Autodesk Inventor part; units mm, degrees
ref_plane "YZ Plane" through (0, 0, 0) normal (1, 0, 0) x (0, 1, 0)
ref_plane "XZ Plane" through (0, 0, 0) normal (0, 1, 0) x (-1, 0, 0)
ref_plane "XY Plane" through (0, 0, 0) normal (0, 0, 1) x (1, 0, 0)
sketch "Sketch1" plane through (0, 0, 0) normal (0, 0, 1) x (1, 0, 0)
  arc A0 (1.778, -29.9361) -> (-1.778, -29.9361) centre (0, -31.75) ccw construction
  line L0 (1.778, -29.9361) -> (1.778, -33.5639) construction
  arc A1 (-1.778, -33.5639) -> (1.778, -33.5639) centre (0, -31.75) ccw construction
  line L1 (-1.778, -33.5639) -> (-1.778, -29.9361) construction
  line L2 (1.778, -29.9361) -> (1.778, -33.5639) construction
  line L3 (-1.778, -29.9361) -> (-1.778, -33.5639) construction
  arc A2 (1.778, -29.9361) -> (-1.778, -29.9361) centre (0, -31.75) ccw construction
  arc A3 (-1.778, -33.5639) -> (1.778, -33.5639) centre (0, -31.75) ccw construction
  arc A4 (1.524, -30.0461) -> (-1.524, -30.0461) centre (0, -31.75) ccw
  line L4 (1.524, -30.0461) -> (1.524, -33.4539)
  arc A5 (-1.524, -33.4539) -> (1.524, -33.4539) centre (0, -31.75) ccw
  line L5 (-1.524, -33.4539) -> (-1.524, -30.0461)
  point P0 (0, 0)
  point P1 (0, -34.29)
  point P2 (0, -29.21)
  dimension "d0" = 0.254
extrude "Extrusion1" add sketch "Sketch1" along normal mid plane 36.83
ref_plane "Work Plane1" through (0, 0, 0) normal (0, 0, 1) x (1, 0, 0)
sketch "Sketch2" plane through (0, 0, 0) normal (0, 0, 1) x (1, 0, 0)
  line L0 (31.75, -50.8) -> (-31.75, -50.8)
  line L1 (-31.75, -50.8) -> (-31.75, -12.7)
  line L2 (-31.75, -12.7) -> (31.75, -12.7)
  line L3 (31.75, -12.7) -> (31.75, -50.8)
  line L4 (31.75, -50.8) -> (-31.75, -12.7) construction
  line L5 (-31.75, -50.8) -> (31.75, -12.7) construction
  circle A0 centre (0, -31.75) radius 5.715
  dimension "d5" = 63.5
  dimension "d6" = 38.1
extrude "Extrusion2" add sketch "Sketch2" along normal mid plane 18.669 contours L0 L1 L2 L3 | A0
properties part number "Geared_Motor"
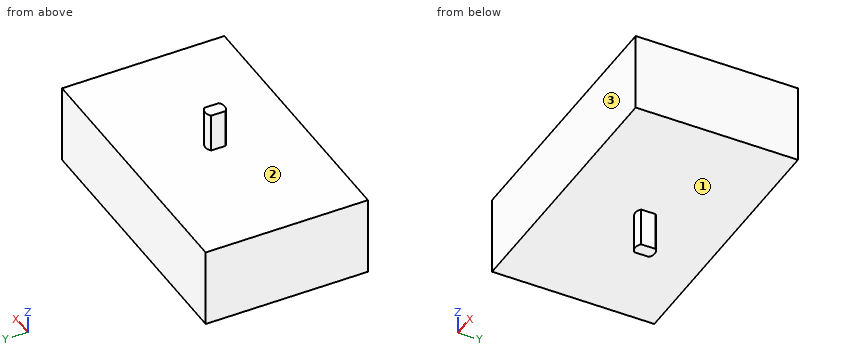
The model under review builds one solid part; all positions refer to its coordinate system, in mm. Face numbers are marked on the shaded views. Round coordinates to 2 decimals unless told otherwise and drop trailing zeros. Write each loop counter-clockwise with the first axis right and the second up, starting at its lowest first coordinate (ties: lowest second). Pieces come first, ordered by that corner, then holes. Notation, with made-up numbers: (37, -39) - (89, -39) arc R34 ccw to (89, -8) - close; hole circle Ø2 at (-38.75, 76.25). An arc over 180 degrees is marked (long way). One line per item, written item: value. Start each with the question number.
1. Consider section B-B on y = -22. Write out the cut boundary in (x, z).
2. Consider section A-A on z = 11.5. Write out the cut boundary in (x, y), and give its area (3 significant figures).
3. Clearance check with flat-ended pins moving along their axes: P1, Ø3.5, axis at y = -32, z = -11.5, coming from the +X side; P2, Ø1.5, axis at x = 5, y = -42, coming from the +Z side; P3, Ø1, axis at y = -31.5, z = 16, coming from the -X side. State where each tip first meets the part, or that it passes through.
4. To check wall thickness, follow L1, parallel to Z at x = 23.5, y = -14.5. State the ranges of the line that lie inside material, in increasing order. Write a range as from..to.
5. The part is to be moulded in two halves that separate along Z. For the marked faces 1, 2 and 3, say which applies: released by +Z, released by -Z, zero draft, split by the parting line, or undercut.
Checks:
1. outline: (-31.75, -9.33) - (31.75, -9.33) - (31.75, 9.33) - (-31.75, 9.33) - close
2. outline: (-1.52, -33.45) arc R2.29 ccw to (1.52, -33.45) - (1.52, -30.05) arc R2.29 ccw to (-1.52, -30.05) - close
2. area: 12.8 mm^2
3. P1: stops at x = 1.52
3. P2: stops at z = 9.33
3. P3: stops at x = -1.52
4. L1: z = -9.33..9.33
5. face 1: released by -Z
5. face 2: released by +Z
5. face 3: zero draft
